Source: CAD feature listing. Evaluate the final solid. Frame: model axes, mm. Face numbers are marked on the shaded views. Give positions to 0.01 mm unless a question says otherwise; leave off trailing zeros. Order: outer loops, then holes, each group sorted by start corner. A loop starts at its lowest first (then second) coordinate and runs counter-clockwise, first axis right, second up. Notation, with made-up numbers: (78.5, 5) - (95.5, 5) arc R22 ccw to (95.5, 18) - close; hole circle Ø8 at (60.25, 38). An arc over 180 degrees is marked (long way). Write each question's results on one line, items separated by ' | '. Start each with the question number.
Item 1: Section D-D on z = 4.75. Output: boundary loops of the cut face in (x, y).
Item 2: Section A-A on y = 11. Output: boundary loops of the cut face in (x, z).
Item 3: Line query: line 1 along Y through (x, z) = (-56.8, 0.4); line 2 along Z through (x, y) = (-32, 3); line 3 along X through (y, z) = (-24.5, 2.75). Output: solid intervals per line, ascending.
Item 4: Contact query for flat-ended pins moving along their axis: pin 1 Ø0.6 at (x, z) = (40.5, -1) entering from -Y; pin 2 Ø5 at (x, y) = (-56.8, 33.8) entering from +Z; pin 3 Ø10 at (x, y) = (-11, -17) entering from -Z; pin 4 Ø2 at (y, z) = (28.5, -0.5) entering from -X. Output: stop coordinate, or through.
Item 5: Section C-C on y = -30.5. Output: boundary loops of the cut face in (x, z).
Item 6: Mould query, pull axis Y, two halves, no side actions, for the marked faces 1 and 2. Classes: released by +Y, released by -Y, zero draft, split by the parting line, or undercut.
Item 7: Section B-B on x = 16. Output: boundary loops of the cut face in (y, z).
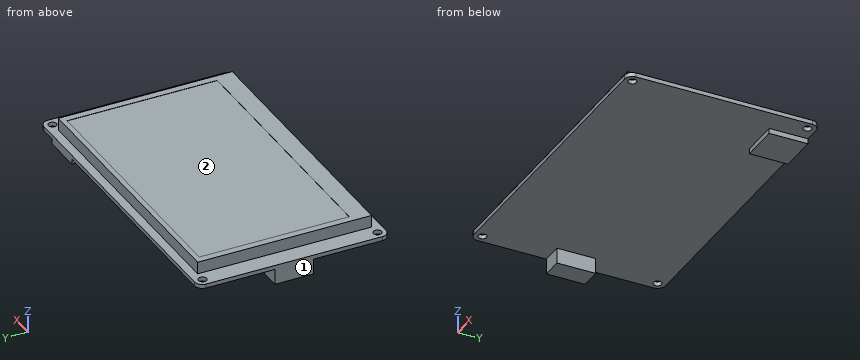
```python
from build123d import *

# Parameters (mm, degrees)
F0_W     = 120
F0_H     = 74
F0_R     = 1.6
F1_DEPTH = 1.6
F2_W     = 105.5
F2_H     = 67.2
F3_DEPTH = 4.7
F4_W     = 100
F4_H     = 58
F5_DEPTH = 0.1
F6_W     = 15
F6_H     = 15
F7_DEPTH = 2
F6_W_2   = 8
F8_DEPTH = 6
F9_R     = 3


with BuildPart() as f1:
    # F0 (on Top) → F1 (new body)
    with BuildSketch(Plane.XY):
        Rectangle(F0_W, F0_H)
        with Locations((-56.8, -33.8)):
            Circle(F0_R, mode=Mode.SUBTRACT)
        with Locations((56.8, -33.8)):
            Circle(F0_R, mode=Mode.SUBTRACT)
        with Locations((-56.8, 33.8)):
            Circle(F0_R, mode=Mode.SUBTRACT)
        with Locations((56.8, 33.8)):
            Circle(F0_R, mode=Mode.SUBTRACT)
    extrude(amount=F1_DEPTH)

    # F2 (on face) → F3 (join)
    with BuildSketch(Plane.XY.offset(1.6)):
        with Locations((0, 0.01)):
            Rectangle(F2_W, F2_H)
    extrude(amount=F3_DEPTH)

    # F4 (on face) → F5 (cut)
    with BuildSketch(Plane.XY.offset(6.3)):
        with Locations((0, 2.61)):
            Rectangle(F4_W, F4_H)
    extrude(amount=-F5_DEPTH, mode=Mode.SUBTRACT)

    # F6 (on face) → F7 (join)
    with BuildSketch(Plane(origin=(0, 0, 0), x_dir=(1, 0, 0), z_dir=(0, 0, -1))):
        with Locations((43.37, -29.5)):
            Rectangle(F6_W, F6_H)
    extrude(amount=F7_DEPTH)

    # F6 (on face) → F8 (join)
    with BuildSketch(Plane(origin=(0, 0, 0), x_dir=(1, 0, 0), z_dir=(0, 0, -1))):
        with Locations((-56, 0)):
            Rectangle(F6_W_2, F6_H)
    extrude(amount=F8_DEPTH)

    # F9
    f9_edges = [f1.edges().sort_by_distance(p)[0] for p in [
        (60, 37, 0.8),
        (60, -37, 0.8),
        (-60, -37, 0.8),
        (-60, 37, 0.8),
    ]]
    fillet(f9_edges, radius=F9_R)


solid = f1.part
```
Evaluation:
1) outline: (-52.75, -33.59) - (52.75, -33.59) - (52.75, 33.61) - (-52.75, 33.61) - close
2) outline: (-60, 0) - (60, 0) - (60, 1.6) - (52.75, 1.6) - (52.75, 6.3) - (50, 6.3) - (50, 6.2) - (-50, 6.2) - (-50, 6.3) - (-52.75, 6.3) - (-52.75, 1.6) - (-60, 1.6) - close
3) line 1: y = -37 to -35.4, -32.2 to 32.2, 35.4 to 37 | line 2: z = 0 to 6.2 | line 3: x = -52.75 to 52.75
4) pin 1: stops at y = 22 | pin 2: stops at z = 1.6 | pin 3: stops at z = 0 | pin 4: stops at x = -60
5) outline: (-60, 0) - (60, 0) - (60, 1.6) - (52.75, 1.6) - (52.75, 6.3) - (-52.75, 6.3) - (-52.75, 1.6) - (-60, 1.6) - close
6) face 1: zero draft | face 2: undercut
7) outline: (-37, 0) - (37, 0) - (37, 1.6) - (33.61, 1.6) - (33.61, 6.3) - (31.61, 6.3) - (31.61, 6.2) - (-26.39, 6.2) - (-26.39, 6.3) - (-33.59, 6.3) - (-33.59, 1.6) - (-37, 1.6) - close
